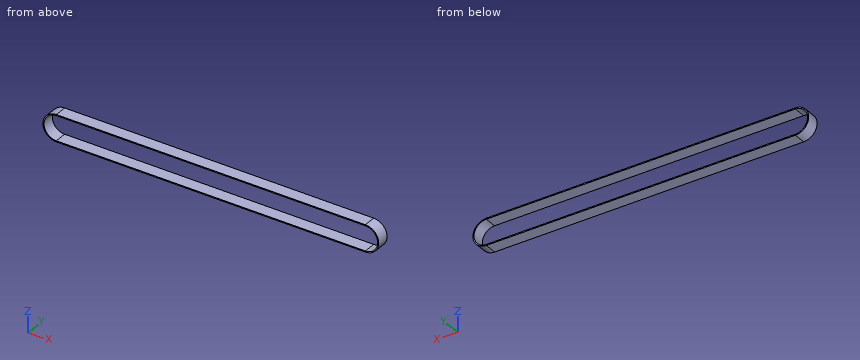
Autodesk Inventor part; units mm, degrees
ref_plane "YZ Plane" through (0, 0, 0) normal (1, 0, 0) x (0, 1, 0)
ref_plane "XZ Plane" through (0, 0, 0) normal (0, 1, 0) x (-1, 0, 0)
ref_plane "XY Plane" through (0, 0, 0) normal (0, 0, 1) x (1, 0, 0)
sketch "スケッチ1" plane through (0, 0, 0) normal (0, 1, 0) x (-1, 0, 0)
  line L0 (75, 6.5) -> (-75, 6.5)
  line L1 (-75, -6.5) -> (75, -6.5)
  line L2 (0, -9.1) -> (0, 9.1)
  line L3 (75, 6.5) -> (75, -6.5) construction
  line L4 (-75, 6.5) -> (-75, -6.5) construction
  circle A0 centre (75, 0) radius 6.5
  circle A1 centre (-75, 0) radius 6.5
  circle A2 centre (75, 0) radius 6
  circle A3 centre (-75, 0) radius 6
  line L5 (75, -6) -> (-75, -6)
  line L6 (-75, 6) -> (75, 6)
  point P0 (0, 0)
  point P1 (75, 6.5)
  point P2 (-75, 6.5)
  dimension "d3" = 13
  dimension "d2" = 150
  dimension "d4" = 12
  dimension "d5" = 12
extrude "押し出し1" add sketch "スケッチ1" along normal blind 6 contours A0 L6 L2 L0 | A0 L5 A2 L6 | L2 L6 A1 L0 | A1 L6 A3 L5 | L1 L2 L5 A0 | A1 L5 L2 L1 picked at (80.8664, -2.29) picked at (-77.4549, -5.7931)
properties part number "belt"
Could you check a few things on this model? Use its own coordinates, in mm. Coordinates: 2 decimals unless noted, no trailing zeros. Order: outer loops, then holes, each group sorted by start corner. A loop starts at its lowest first (then second) coordinate and runs counter-clockwise, first axis right, second up. Notation, with made-up numbers: M 36,-39 L 63,-39 A21 ccw 63,-21 Z; hole C 29.5,-33 d2. An arc over 180 degrees is marked long. Use one line per item in the form item = value. Start each with the question number.
1. Suppose I cut it at B-B on y = 3. Write out the boundary of the cut face in (x, z), then the cut area to 3 significant figures.
2. For pin 1 (1.5 mm diameter, centred on y = 3.5, z = 1, fed in from -X); pin 2 (5 mm diameter, centred on x = 0.5, z = 3, fed in from +Y), each with a flat end and sliding along its axis, tell me the tip position at first contact or that it passes through.
3. Please list where these lines run through material, in increasing order: line 1 (Z direction, x = 10, y = 0.3); line 2 (X direction, y = 0.35, z = -0.5); line 3 (X direction, y = 0.4, z = -4.25).
4. Suppose I cut it at C-C on x = 10. Write out the boundary of the cut face in (y, z), then the cut area to 3 significant figures.
5. Suppose I cut it at A-A on z = 0. Write out the boundary of the cut face in (x, y).
Geometry says:
q1.outline = M -75,-6.5 L 75,-6.5 A6.5 ccw 75,6.5 L -75,6.5 A6.5 ccw Z; hole M -75,-6 L 75,-6 A6 ccw 75,6 L -75,6 A6 ccw Z
q1.area = 170 mm^2
q2.pin_1 = -81.5
q2.pin_2 = through
q3.line_1 = -6.5 to -6, 6 to 6.5
q3.line_2 = -81.48 to -80.98, 80.98 to 81.48
q3.line_3 = -79.92 to -79.24, 79.24 to 79.92
q4.outline = M 0,-6.5 L 6,-6.5 L 6,-6 L 0,-6 Z; M 0,6 L 6,6 L 6,6.5 L 0,6.5 Z
q4.area = 6.00 mm^2
q5.outline = M -81.5,0 L -81,0 L -81,6 L -81.5,6 Z; M 81,0 L 81.5,0 L 81.5,6 L 81,6 Z
